Geometry check sheet. Reference: the model listing, model coordinates, mm. A direction names the side the tool comes from. Give positions to 0.01 mm unless a question says otherwise; leave off trailing zeros. Write each loop counter-clockwise with the first axis right and the second up, starting at its lowest first coordinate (ties: lowest second). Pieces come first, ordered by that corner, then holes.
(1) Tool access check on faces 1 (the flat face through (-271, 245, -26)), 2 (the flat face through (-271, 295, -26)), 3 (the flat face through (269, -245, 20)), 4 (the flat face through (269, -295, 20)). Record the directions out of +Z, -Z, +X, -X, +Y, -Y that give a thin tool (end or side, any length) a straight path to the whole face; none if there is none.
(2) Cross-section at A-A (z = -15). Record the boundary of the cut face in (x, y), and give its area (3 significant figures).
(3) Cross-section at B-B (x = -270). Record the boundary of the cut face in (y, z), and give its area (3 significant figures).
(4) Depth check by flat-ended pin: P1, Ø21, axis at x = 274, z = 25.5, coming from the -Y side; P2, Ø8, axis at x = 152, z = 17, coming from the +Y side; P3, Ø1, axis at x = 182.5, y = -105, coming from the -Z side; P4, Ø2, axis at x = -148.5, y = -133, coming from the +Z side. Enter the tip coordinate at first touch or a pass-through.
(5) Cross-section at C-C (z = 23). Record the boundary of the cut face in (x, y).
(6) Thickness scan on line 1 along Y through (x, z) = (313.5, -31.5); line 2 along Z through (x, y) = (29, 207); line 3 along X through (y, z) = (264.5, -29.5). Record the ranges inside material, lowest first.
(7) Mould release check, pull along Z, two halves, no side actions. Record for faces 5 (the flat face through (269, 295, -26)), 6 (the cylindrical face through (-268.665, -269.65, -65.983)), 7 (the cylindrical face through (269.244, 270.35, 35.994)): +Z half, -Z half, draft (parallel to the pull), parting line (faces both ways), or undercut.
(8) Cross-section at D-D (y = -131.5). Record the boundary of the cut face in (x, z), and give its area (3 significant figures).
```python
from build123d import *

# Parameters (mm, degrees)
SKETCH_1_W      = 700
SKETCH_1_H      = 700
EXTRUDE_1_DEPTH = 10
SKETCH_2_R      = 51
EXTRUDE_2_DEPTH = 25


with BuildPart() as part:
    # 草图1 → 凸台-拉伸1 (new body)
    with BuildSketch(Plane.XY):
        Rectangle(SKETCH_1_W, SKETCH_1_H)
    extrude(amount=EXTRUDE_1_DEPTH)

    # 草图2 → 凸台-拉伸2 (add, symmetric)
    with BuildSketch(Plane(origin=(0, 270, 0), x_dir=(1, 0, 0), z_dir=(0, 1, 0))):
        with Locations((-270, 15)):
            Circle(SKETCH_2_R)
        with Locations((270, 15)):
            Circle(SKETCH_2_R)
    extrude_2 = extrude(amount=EXTRUDE_2_DEPTH, both=True)

    # 镜向1: 凸台-拉伸2 across plane
    add(extrude_2.mirror(Plane.ZX))


solid = part.part
```
Reply:
1. face 1: -Z, +X, -X
1. face 2: -Z, +X, -X, +Y
1. face 3: +Z, +X, -X
1. face 4: +Z, +X, -X, -Y
2. outline: (-321, -295) - (-219, -295) - (-219, -245) - (-321, -245) - close; (-321, 245) - (-219, 245) - (-219, 295) - (-321, 295) - close; (219, -295) - (321, -295) - (321, -245) - (219, -245) - close; (219, 245) - (321, 245) - (321, 295) - (219, 295) - close
2. area: 20,400 mm2
3. outline: (-350, 0) - (-295, 0) - (-295, -66) - (-245, -66) - (-245, 0) - (245, 0) - (245, -66) - (295, -66) - (295, 0) - (350, 0) - (350, 10) - (295, 10) - (295, 36) - (245, 36) - (245, 10) - (-245, 10) - (-245, 36) - (-295, 36) - (-295, 10) - (-350, 10) - close
3. area: 16,200 mm2
4. P1: stops at y = -295
4. P2: passes through
4. P3: stops at z = 0
4. P4: stops at z = 10
5. outline: (-304.01, -295) - (-235.99, -295) - (-235.99, -245) - (-304.01, -245) - close; (-304.01, 245) - (-235.99, 245) - (-235.99, 295) - (-304.01, 295) - close; (235.99, -295) - (304.01, -295) - (304.01, -245) - (235.99, -245) - close; (235.99, 245) - (304.01, 245) - (304.01, 295) - (235.99, 295) - close
6. line 1: y = -295 to -245, 245 to 295
6. line 2: z = 0 to 10
6. line 3: x = -318.9 to -221.1, 221.1 to 318.9
7. face 5: draft
7. face 6: undercut
7. face 7: +Z half
8. outline: (-350, 0) - (350, 0) - (350, 10) - (-350, 10) - close
8. area: 7,000 mm2
